Geometry check sheet. Reference: the model listing, model coordinates, mm. A direction names the side the tool comes from. Round coordinates to 2 decimals unless told otherwise and drop trailing zeros. Write each loop counter-clockwise with the first axis right and the second up, starting at its lowest first coordinate (ties: lowest second). Pieces come first, ordered by that corner, then holes.
from build123d import *

# Parameters (mm, degrees)
BOSS_EXTRUDE1_DEPTH = 127


with BuildPart() as part:
    # Sketch1 → Boss-Extrude1 (new body)
    with BuildSketch(Plane(origin=(0, 0, 0), x_dir=(1, 0, 0), z_dir=(0, 1, 0))):
        with BuildLine():
            Line((-231.775, 165.1), (-231.775, -177.8))
            Line((-231.775, -177.8), (-228.6, -177.8))
            Line((-228.6, -177.8), (-228.6, 165.1))
            ThreePointArc((-228.6, 165.1), (-224.880256121, 174.080256121), (-215.9, 177.8))
            Line((-215.9, 177.8), (215.9, 177.8))
            ThreePointArc((215.9, 177.8), (224.880256121, 174.080256121), (228.6, 165.1))
            Line((228.6, 165.1), (228.6, -177.8))
            Line((228.6, -177.8), (231.775, -177.8))
            Line((231.775, -177.8), (231.775, 165.1))
            ThreePointArc((231.775, 165.1), (227.125320151, 176.325320151), (215.9, 180.975))
            Line((215.9, 180.975), (-215.9, 180.975))
            ThreePointArc((-215.9, 180.975), (-227.125320151, 176.325320151), (-231.775, 165.1))
        make_face()
    extrude(amount=BOSS_EXTRUDE1_DEPTH)


solid = part.part
1. Section check A-A (z = 152). Record the cut outline in (x, y) (3 decimals).
2. Section check C-C (x = 112.5). Record the cut outline in (y, z) (3 decimals), plus the area to 3 significant figures.
3. Access from +Z, -Z, +X, -X, +Y, -Y to the whole of each face (thin tool, end or side, straight path). Record for faces 1 (the face through (231.775, 63, 9)), 2 (the face through (-3, 63, -177.8)).
4. Section check B-B (y = 33). Record the cut outline in (x, z) (3 decimals), plus the area to 3 significant figures.
5. Depth check by flat-ended pin: pin 1 Ø10 at (x, y) = (-151, 78) entering from +Z. Enter the tip coordinate at first touch or a pass-through.
6. Release check for a two-part mould opening along X. For faces 3 (the face through (227.25, 62.61, -176.2)), 4 (the face through (3, 63, -180.975)), 5 (the face through (228.6, 63, 4)) record: +X half, -X half, draft (parallel to the pull), parting line (faces both ways), or undercut.
7. Scan lines: line 1 along X through (y, z) = (42, -66.5) (3 decimals); line 2 along Z through (x, y) = (209.5, 26) (3 decimals). Record each from-to range of solid material in increasing order.
Results below:
1. outline: (-231.775, 0) - (-228.6, 0) - (-228.6, 127) - (-231.775, 127) - close; (228.6, 0) - (231.775, 0) - (231.775, 127) - (228.6, 127) - close
2. outline: (0, -180.975) - (127, -180.975) - (127, -177.8) - (0, -177.8) - close
2. area: 403 mm2
3. face 1: +Z, -Z, +X, +Y, -Y
3. face 2: +Z, +Y, -Y
4. outline: (-231.775, -165.1) arc R15.875 ccw to (-215.9, -180.975) - (215.9, -180.975) arc R15.875 ccw to (231.775, -165.1) - (231.775, 177.8) - (228.6, 177.8) - (228.6, -165.1) arc R12.7 cw to (215.9, -177.8) - (-215.9, -177.8) arc R12.7 cw to (-228.6, -165.1) - (-228.6, 177.8) - (-231.775, 177.8) - close
4. area: 3,690 mm2
5. pin 1: stops at z = -177.8
6. face 3: +X half
6. face 4: draft
6. face 5: undercut
7. line 1: x = -231.775 to -228.6, 228.6 to 231.775
7. line 2: z = -180.975 to -177.8
